```python
from build123d import *

# Parameters (mm, degrees)
SKETCH1_R           = 3
BOSS_EXTRUDE1_DEPTH = 4
FILLET1_R           = 3
FILLET2_R           = 3
BOSS_EXTRUDE2_START = -2
BOSS_EXTRUDE2_DEPTH = 2
SKETCH2_R           = 2.5
CUT_EXTRUDE1_DEPTH  = 29.372521918
SKETCH4_R           = 0.9
BOSS_EXTRUDE3_DEPTH = 3


with BuildPart() as part:
    # Sketch1 → Boss-Extrude1 (new body)
    with BuildSketch(Plane.XY):
        with BuildLine():
            Line((3.494878983, 2.834752351), (1.063186177, 5.732879237))
            ThreePointArc((1.063186177, 5.732879237), (-0.407640956, 6.688232403), (-2.161242517, 6.658005015))
            ThreePointArc((-2.161242517, 6.658005015), (-6.541414145, -2.491967293), (2.816438132, -6.408406686))
            ThreePointArc((2.816438132, -6.408406686), (4.145674153, -5.264219757), (4.608056658, -3.572405775))
            Line((4.608056658, -3.572405775), (4.495140924, 0.209064756))
            Line((4.495140924, 0.209064756), (17.788851391, 5.614937189))
            ThreePointArc((17.788851391, 5.614937189), (24.73795094, 9.42398131), (17.01587301, 7.64400544))
            Line((17.01587301, 7.64400544), (3.494878983, 2.834752351))
        make_face()
        with Locations((21, 8)):
            Circle(SKETCH1_R, mode=Mode.SUBTRACT)
    extrude(amount=BOSS_EXTRUDE1_DEPTH)

    # Fillet1
    fillet1_edges = [part.edges().sort_by_distance(p)[0] for p in [
        (3.494878983, 2.834752351, 2),
        (4.495140924, 0.209064756, 2),
    ]]
    fillet(fillet1_edges, radius=FILLET1_R)

    # Fillet2
    fillet2_edges = [part.edges().sort_by_distance(p)[0] for p in [
        (17.01587301, 7.64400544, 2),
        (17.788851391, 5.614937189, 2),
    ]]
    fillet(fillet2_edges, radius=FILLET2_R)

    # Sketch1_3 → Boss-Extrude2 (add)
    with BuildSketch(Plane.XY.offset(BOSS_EXTRUDE2_START)):
        with BuildLine():
            Line((3.398714044, 2.949363125), (1.063186177, 5.732879237))
            ThreePointArc((1.063186177, 5.732879237), (-0.407640956, 6.688232403), (-2.161242517, 6.658005015))
            ThreePointArc((-2.161242517, 6.658005015), (-6.541414145, -2.491967293), (2.816438132, -6.408406686))
            ThreePointArc((2.816438132, -6.408406686), (4.145674153, -5.264219757), (4.608056658, -3.572405775))
            Line((4.608056658, -3.572405775), (4.499606346, 0.059520833))
            ThreePointArc((4.499606346, 0.059520833), (4.205194807, 1.601978974), (3.398714044, 2.949363125))
        make_face()
    extrude(amount=BOSS_EXTRUDE2_DEPTH)

    # Sketch2 → Cut-Extrude1 (cut, through all)
    with BuildSketch(Plane.XY.offset(4)):
        Circle(SKETCH2_R)
    extrude(amount=-CUT_EXTRUDE1_DEPTH, mode=Mode.SUBTRACT)

    # Sketch4 → Boss-Extrude3 (add)
    with BuildSketch(Plane.XY.offset(-2)):
        with Locations((-2.135971966, 5.60692641)):
            Circle(SKETCH4_R)
        with Locations(Location((2.135971966, -5.60692641, 0), (0, 0, 180))):
            Circle(SKETCH4_R)
        with Locations(Location((-5.60692641, -2.135971966, 0), (0, 0, 180))):
            Circle(SKETCH4_R)
    extrude(amount=-BOSS_EXTRUDE3_DEPTH)


solid = part.part
```
Could you check a few things on this model? Use its own coordinates, in mm. A direction names the side the tool comes from. Coordinates: 2 decimals unless noted, no trailing zeros. Write each loop counter-clockwise with the first axis right and the second up, starting at its lowest first coordinate (ties: lowest second). Pieces come first, ordered by that corner, then holes. Notation, with made-up numbers: (24.5, 54.5) - (66.5, 54.5) arc R9 ccw to (66.5, 70.5) - close; hole circle Ø11 at (-20.75, 79). An arc over 180 degrees is marked (long way). Use a Markdown table: item, result.
Q1. Imagine slicing it at C-C (y = 8). List the corners of the cut face in (x, z) for me, and give its area (3 significant figures).
Geometry check:
| item | result |
|---|---|
| outline | (16.61, 0) - (18, 0) - (18, 4) - (16.61, 4) - close; (24, 0) - (25, 0) - (25, 4) - (24, 4) - close |
| area | 9.54 mm2 |
Q2. Which directions (+Z, -Z, +X, -X, +Y, -Y) give clear straight access to the entire face, cutting with the end or side of a thin tool? Please do faces 1 (the flat face through (11.173, 2.925, 1.972)), 2 (the cylindrical face through (-4.71, -2.18, -3.48)), 3 (the cylindrical face through (-0.38, 6.68, 0.96)), 4 (the cylindrical face through (4.213, 1.581, -1.014)).
Geometry check:
| item | result |
|---|---|
| face 1 | +Z, -Z, -Y |
| face 2 | -Z |
| face 3 | +Z, -Z, +Y |
| face 4 | -Z, +X, +Y |
Q3. Please list where these lines run through material, in increasing order: L1, parallel to Y at x = 21, z = 2.45; L2, parallel to Z at x = 16, y = 7; L3, parallel to X at y = 1.75, z = 3.5.
Geometry check:
| item | result |
|---|---|
| L1 | y = 4 to 5, 11 to 12 |
| L2 | z = 0 to 4 |
| L3 | x = -6.78 to -1.79, 1.79 to 8.28 |
Q4. Thinking about a two-plate mould opening in Y: for faces 5 (the cylindrical face through (-1.72, 4.81, -3.48)), 6 (the cylindrical face through (18, 8, 2)), 7 (the flat face through (2, -6, -5)), 8 (the cylindrical face through (5.056, -0.126, 2.028)), which applies, +Y half, -Y half, draft (parallel to the pull), parting line (faces both ways), or undercut?
Geometry check:
| item | result |
|---|---|
| face 5 | parting line |
| face 6 | undercut |
| face 7 | draft |
| face 8 | undercut |
Q5. Imagine slicing it at D-D (z = -4). List the corners of the cut face in (x, y) for me.
Geometry check:
| item | result |
|---|---|
| outline | circle Ø1.8 at (-5.61, -2.14); circle Ø1.8 at (-2.14, 5.61); circle Ø1.8 at (2.14, -5.61) |
Q6. Imagine slicing it at A-A (x = 21). List the corners of the cut face in (y, z) for me, and give its area (3 significant figures).
Geometry check:
| item | result |
|---|---|
| outline | (4, 0) - (5, 0) - (5, 4) - (4, 4) - close; (11, 0) - (12, 0) - (12, 4) - (11, 4) - close |
| area | 8.00 mm2 |
Q7. I'm going to push flat-ended pins straight in: pin 1 Ø8 at (x, y) = (9.5, -0.5) entering from +Z; pin 2 Ø4 at (y, z) = (6, -2.5) entering from -X; pin 3 Ø4 at (x, z) = (12.5, 0.5) entering from +Y; pin 4 Ø9.5 at (x, y) = (21, 8) entering from -Z. Where does each tip first touch, or does it pass through?
Geometry check:
| item | result |
|---|---|
| pin 1 | stops at z = 4 |
| pin 2 | stops at x = -5.7 |
| pin 3 | stops at y = 6.75 |
| pin 4 | stops at z = 0 |
Q8. Imagine slicing it at B-B (z = 2). List the corners of the cut face in (x, y) for me (3 decimals), and give its area (3 significant figures).
Geometry check:
| item | result |
|---|---|
| outline | (-2.161, 6.658) arc R7 ccw (long way) to (2.816, -6.408) arc R3 ccw to (4.608, -3.572) - (4.557, -1.874) arc R3 cw to (6.426, 0.994) - (16.055, 4.91) arc R3 cw to (18.82, 4.646) arc R4 ccw (long way) to (17.141, 9.053) arc R3 cw to (15.252, 7.017) - (5.459, 3.533) arc R3 cw to (2.155, 4.431) - (1.063, 5.733) arc R3 ccw to start; hole circle Ø5 at (0, 0); hole circle Ø6 at (21, 8) |
| area | 165 mm2 |
